Source: CAD feature listing. Evaluate the final solid. Frame: model axes, mm. Face numbers are marked on the shaded views. A direction names the side the tool comes from. Round coordinates to 2 decimals unless told otherwise and drop trailing zeros. Order: outer loops, then holes, each group sorted by start corner. A loop starts at its lowest first (then second) coordinate and runs counter-clockwise, first axis right, second up. Notation, with made-up numbers: (-2, -3) - (41, -3) arc R19 cw to (41, 25) - close; hole circle Ø1 at (-38.5, 55.5). An arc over 180 degrees is marked (long way). Use one line per item in the form item = value. Start each with the question number.
Q1. Cut plane B-B, the plane y = -15.24. Return the cut outline in (x, z), and give its area (3 significant figures).
Q2. Pin query (flat end, axial travel): pin 1 Ø4 at (y, z) = (-19.5, -1) entering from +X; pin 2 Ø6 at (x, y) = (-3, -15.5) entering from -Z; pin 3 Ø6 at (x, y) = (4.5, -19) entering from -Z; pin 4 Ø5 at (x, y) = (-2, -19.5) entering from +Z. Return the tip coordinate at first contact, or that it passes through.
Q3. Set-up query: the marked faces 5, 6 and 7. Return all of +Z, -Z, +X, -X, +Y, -Y with unobstructed straight access to the full face (end or side cutting, diameter ignored); none if empty.
Q4. Cut plane C-C, the plane z = -8. Return the cut outline in (x, y), and give its area (3 significant figures).
Q5. Cut plane A-A, the plane z = -0.5. Return the cut outline in (x, y), and give its area (3 significant figures).
Q6. Cut plane D-D, the plane x = 1.5. Return the cut outline in (y, z), and give its area (3 significant figures).
Q7. Ray query, line 1 (Y direction, x = -0.25, z = 6.5); line 2 (Y direction, x = -1.75, z = 0); line 3 (X direction, y = -12.25, z = -6.5). Return the intervals inside material, ascending. Write a range as [from, to].
Q8. Draft query along X for the marked faces 1, 2, 3 and 4. Return one class per face: released by +X, released by -X, zero draft, split by the parting line, or undercut.
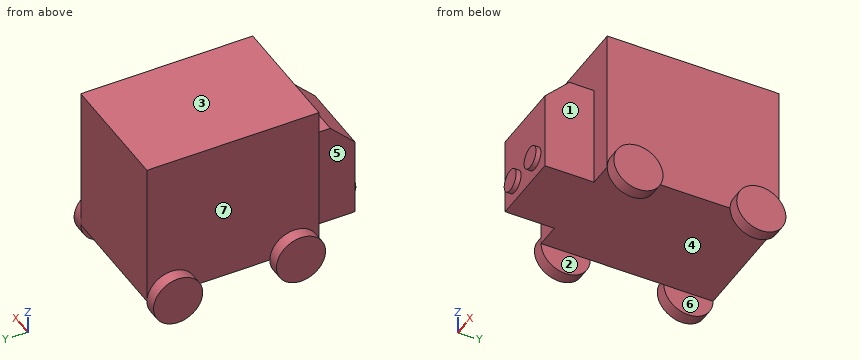
from build123d import *

# Parameters (mm, degrees)
F0_W     = 12.7
F0_H     = 15.24
F1_DEPTH = 17.78
F3_DEPTH = 5.08
F5_DEPTH = 1.27
F7_DEPTH = 0.508
F9_DEPTH = 1.27
F10_SIZE = 2.54


with BuildPart() as f1:
    # F0 (on Front) → F1 (new body)
    with BuildSketch(Plane.XZ):
        Rectangle(F0_W, F0_H)
    extrude(amount=F1_DEPTH)

    # F2 (on face) → F3 (join)
    with BuildSketch(Plane.XZ.offset(17.78)):
        Polygon((3.81, 3.048), (-3.81, 3.048), (-3.81, -7.62), (3.8175627124, -7.62), (3.8175627124, 3.048), align=None)
    extrude(amount=F3_DEPTH)

    # F4 (on face) → F5 (join)
    with BuildSketch(Plane(origin=(-6.35, 0, 0), x_dir=(0, -1, 0), z_dir=(-1, 0, 0))):
        with BuildLine():
            Line((0, -7.62), (5.08, -7.62))
            ThreePointArc((5.08, -7.62), (2.54, -5.08), (0, -7.62))
        make_face()
        with BuildLine():
            ThreePointArc((0, -7.62), (2.54, -10.16), (5.08, -7.62))
            Line((5.08, -7.62), (0, -7.62))
        make_face()
        with BuildLine():
            Line((12.7, -7.62), (17.78, -7.62))
            ThreePointArc((17.78, -7.62), (15.24, -5.08), (12.7, -7.62))
        make_face()
        with BuildLine():
            ThreePointArc((12.7, -7.62), (15.24, -10.16), (17.78, -7.62))
            Line((17.78, -7.62), (12.7, -7.62))
        make_face()
    extrude(amount=F5_DEPTH)

    # F6 (on face) → F7 (join)
    with BuildSketch(Plane.XZ.offset(22.86)):
        with BuildLine():
            Line((-3.0461093219, -5.4919943213), (-0.7601093219, -5.4919943213))
            ThreePointArc((-0.7601093219, -5.4919943213), (-1.9031093219, -4.3489943213), (-3.0461093219, -5.4919943213))
        make_face()
        with BuildLine():
            ThreePointArc((-3.0461093219, -5.4919943213), (-1.9031093219, -6.6349943213), (-0.7601093219, -5.4919943213))
            Line((-0.7601093219, -5.4919943213), (-3.0461093219, -5.4919943213))
        make_face()
        with BuildLine():
            ThreePointArc((3.0536720343, -5.4919943213), (1.9106720343, -4.3489943213), (0.7676720343, -5.4919943213))
            Line((0.7676720343, -5.4919943213), (3.0536720343, -5.4919943213))
        make_face()
        with BuildLine():
            Line((3.0536720343, -5.4919943213), (0.7676720343, -5.4919943213))
            ThreePointArc((0.7676720343, -5.4919943213), (1.9106720343, -6.6349943213), (3.0536720343, -5.4919943213))
        make_face()
    extrude(amount=F7_DEPTH)

    # F8 (on face) → F9 (join)
    with BuildSketch(Plane.YZ.offset(6.35)):
        with BuildLine():
            ThreePointArc((-17.78, -7.62), (-15.24, -10.16), (-12.7, -7.62))
            Line((-12.7, -7.62), (-17.78, -7.62))
        make_face()
        with BuildLine():
            Line((-17.78, -7.62), (-12.7, -7.62))
            ThreePointArc((-12.7, -7.62), (-15.24, -5.08), (-17.78, -7.62))
        make_face()
        with BuildLine():
            ThreePointArc((0, -7.62), (-2.54, -5.08), (-5.08, -7.62))
            Line((-5.08, -7.62), (0, -7.62))
        make_face()
        with BuildLine():
            Line((0, -7.62), (-5.08, -7.62))
            ThreePointArc((-5.08, -7.62), (-2.54, -10.16), (0, -7.62))
        make_face()
    extrude(amount=F9_DEPTH)

    # F10
    f10_edges = [f1.edges().sort_by_distance(p)[0] for p in [
        (0.003781, -22.86, 3.048),
    ]]
    chamfer(f10_edges, length=F10_SIZE)


solid = f1.part
Completed:
q1.outline = (-7.62, -10.16) - (-6.35, -10.16) - (-6.35, -7.62) - (6.35, -7.62) - (6.35, -10.16) - (7.62, -10.16) - (7.62, -5.08) - (6.35, -5.08) - (6.35, 7.62) - (-6.35, 7.62) - (-6.35, -5.08) - (-7.62, -5.08) - close
q1.area = 206 mm2
q2.pin_1 = 6.35
q2.pin_2 = -7.62
q2.pin_3 = -9.74
q2.pin_4 = 7.62
q3.face_5 = +Z, -Z, -X, -Y
q3.face_6 = -Z, +Y, -Y
q3.face_7 = +Z, -X
q4.outline = (-7.62, -17.75) - (-6.35, -17.75) - (-6.35, -12.73) - (-7.62, -12.73) - close; (-7.62, -5.05) - (-6.35, -5.05) - (-6.35, -0.03) - (-7.62, -0.03) - close; (6.35, -17.75) - (7.62, -17.75) - (7.62, -12.73) - (6.35, -12.73) - close; (6.35, -5.05) - (7.62, -5.05) - (7.62, -0.03) - (6.35, -0.03) - close
q4.area = 25.5 mm2
q5.outline = (-6.35, -17.78) - (-3.81, -17.78) - (-3.81, -22.86) - (3.82, -22.86) - (3.82, -17.78) - (6.35, -17.78) - (6.35, 0) - (-6.35, 0) - close
q5.area = 265 mm2
q6.outline = (-23.37, -6.56) - (-22.86, -6.56) - (-22.86, -7.62) - (0, -7.62) - (0, 7.62) - (-17.78, 7.62) - (-17.78, 3.05) - (-20.32, 3.05) - (-22.86, 0.51) - (-22.86, -4.43) - (-23.37, -4.43) - close
q6.area = 323 mm2
q7.line_1 = [-17.78, 0]
q7.line_2 = [-22.86, 0]
q7.line_3 = [-6.35, 6.35]
q8.face_1 = released by +X
q8.face_2 = undercut
q8.face_3 = zero draft
q8.face_4 = undercut
